Read the model definition and answer for the solid it produces. Units are mm, in the model's axes. A direction names the side the tool comes from. Coordinates: 2 decimals unless noted, no trailing zeros. Write each loop counter-clockwise with the first axis right and the second up, starting at its lowest first coordinate (ties: lowest second). Pieces come first, ordered by that corner, then holes.
Item 1: Straight lines are drawn through the part: probe 1 along Z at (x, y) = (0, 7.5); probe 2 along Y at (x, z) = (0, 4.6) (3 decimals). For each, find the intervals that lie inside material, in ascending order.
Item 2: Each of these flat-tipped pins is pushed along its axis until it touches: P1, Ø3, axis at x = -1, y = 12.5, coming from the +Z side; P2, Ø5, axis at x = 1, y = 13.5, coming from the -Z side; P3, Ø7.5, axis at y = 16.5, z = -1.5, coming from the +X side; P4, Ø3, axis at x = 0, y = 14.29, coming from the -Z side. Where does it stop, or does it pass through?
Item 3: Section C-C (x = 0) is taken. State how many separate pieces and enclosed holes the cut face has, then the cut area to 3 significant figures.
Item 4: A tool of negligible diameter and unlimited length cuts with its end or side. For faces 1 (the face through (-6.35, 13, 0)), 2 (the face through (6.35, 13, 0)), 3 (the face through (5.9, 13.12, -5.87)), 4 (the face through (0, 11, -6.35)), from which of +Z, -Z, +X, -X, +Y, -Y can it reach the whole face along a straight path? Write none if from no direction.
Item 5: Determine the mould class of faces 5 (the face through (0.067, 3.628, -6.827)), 6 (the face through (5.87, 13.12, 5.9)), 7 (the face through (1.647, 7.494, -0.519)) for opening direction X: released by +X, released by -X, zero draft, split by the parting line, or undercut.
Item 6: Section A-A (y = 8.5) is taken. Give the vertices of the cut face in (x, z), then the cut area to 3 significant figures.
from build123d import *

# Parameters (mm, degrees)
SKETCH1_W             = 19.05
SKETCH1_H             = 19.05
BOSS_EXTRUDE1_DEPTH   = 22.225
SKETCH2_OUTSIDE_W     = 28.034
SKETCH2_OUTSIDE_H     = 28.034
SKETCH2_OUTSIDE_W_2   = 12.7
SKETCH2_OUTSIDE_H_2   = 12.7
CUT_EXTRUDE1_DEPTH    = 19.05
F_8_32_TAPPED_HOLE2_D = 3.4544
F_8_32_TAPPED_HOLE1_D = 3.4544
FILLET1_R             = 1.5875
CHAMFER1_SIZE         = 0.508


with BuildPart() as part:
    # Sketch1 → Boss-Extrude1 (new body)
    with BuildSketch(Plane(origin=(0, 0, 0), x_dir=(1, 0, 0), z_dir=(0, 1, 0))):
        Rectangle(SKETCH1_W, SKETCH1_H)
    extrude(amount=BOSS_EXTRUDE1_DEPTH)

    # Sketch2 outside → Cut-Extrude1 (cut)
    with BuildSketch(Plane(origin=(0, 22.225, 0), x_dir=(1, 0, 0), z_dir=(0, 1, 0))):
        Rectangle(SKETCH2_OUTSIDE_W, SKETCH2_OUTSIDE_H)
        Rectangle(SKETCH2_OUTSIDE_W_2, SKETCH2_OUTSIDE_H_2, mode=Mode.SUBTRACT)
    extrude(amount=-CUT_EXTRUDE1_DEPTH, mode=Mode.SUBTRACT)

    # #8-32 Tapped Hole2 (through all)
    with Locations(Plane(origin=(0, 0, 0), x_dir=(-1, 0, 0), z_dir=(0, -1, 0))):
        with Locations((0, 0)):
            Hole(F_8_32_TAPPED_HOLE2_D / 2)

    # #8-32 Tapped Hole1 (through all)
    with Locations(Plane.XY.offset(6.35)):
        with Locations((0, 14.2875)):
            Hole(F_8_32_TAPPED_HOLE1_D / 2)

    # Fillet1
    fillet1_edges = [part.edges().sort_by_distance(p)[0] for p in [
        (9.525, 1.5875, 9.525),
        (-9.525, 1.5875, 9.525),
        (-9.525, 1.5875, -9.525),
        (9.525, 1.5875, -9.525),
        (0, 3.175, 6.35),
        (6.35, 3.175, 0),
        (0, 3.175, -6.35),
        (-6.35, 3.175, 0),
        (6.35, 12.7, 6.35),
        (-6.35, 12.7, 6.35),
        (-6.35, 12.7, -6.35),
        (6.35, 12.7, -6.35),
        (0, 0, 9.525),
        (-9.525, 0, 0),
        (0, 0, -9.525),
        (9.525, 0, 0),
    ]]
    fillet(fillet1_edges, radius=FILLET1_R - 0.0001)  # a hair under: the kernel refuses the full size

    # Chamfer1
    chamfer1_edges = [part.edges().sort_by_distance(p)[0] for p in [
        (-1.7272, 0, 0),
        (-1.7272, 22.225, 0),
        (1.7272, 14.2875, -6.35),
        (1.7272, 14.2875, 6.35),
        (0, 22.225, 6.35),
        (6.35, 22.225, 0),
        (0, 22.225, -6.35),
        (-6.35, 22.225, 0),
        (-5.885061304, 22.225, -5.885061304),
        (5.885061304, 22.225, -5.885061304),
        (-5.885061304, 22.225, 5.885061304),
        (5.885061304, 22.225, 5.885061304),
        (-9.525, 3.175, 0),
        (0, 3.175, 9.525),
        (9.525, 3.175, 0),
        (0, 3.175, -9.525),
        (9.060061304, 3.175, -9.060061304),
        (-9.060061304, 3.175, -9.060061304),
        (-9.060061304, 3.175, 9.060061304),
        (9.060061304, 3.175, 9.060061304),
    ]]
    chamfer(chamfer1_edges, length=CHAMFER1_SIZE)


solid = part.part
Established:
1. probe 1: z = -6.35 to -1.73, 1.73 to 6.35
1. probe 2: y = 0 to 12.56, 16.015 to 22.225
2. P1: stops at z = 6.35
2. P2: stops at z = -6.35
2. P3: stops at x = 6.35
2. P4: passes through
3. separate pieces: 4
3. enclosed holes: 0
3. area: 192 mm2
4. face 1: +Z, -Z, -X, +Y
4. face 2: +Z, -Z, +X, +Y
4. face 3: -Z, +X, +Y
4. face 4: -Z, +X, -X, +Y
5. face 5: zero draft
5. face 6: released by +X
5. face 7: undercut
6. outline: (-6.35, -4.76) arc R1.59 ccw to (-4.76, -6.35) - (4.76, -6.35) arc R1.59 ccw to (6.35, -4.76) - (6.35, 4.76) arc R1.59 ccw to (4.76, 6.35) - (-4.76, 6.35) arc R1.59 ccw to (-6.35, 4.76) - close; hole circle Ø3.45 at (0, 0)
6. area: 150 mm2
